Build history of the part. All positions in model axes, mm. Face numbers are marked on the shaded views. Give positions to 0.01 mm unless a question says otherwise; leave off trailing zeros. Loops run counter-clockwise (first coordinate to the right, second up) from the corner with the lowest first, then second, coordinate; pieces in that order, holes last. Notation, with made-up numbers: M 32,87 L 42,87 A12 cw 42,103 Z; hole C 27.25,-13 d2. An arc over 180 degrees is marked long. Put each result on its own line as item: value.
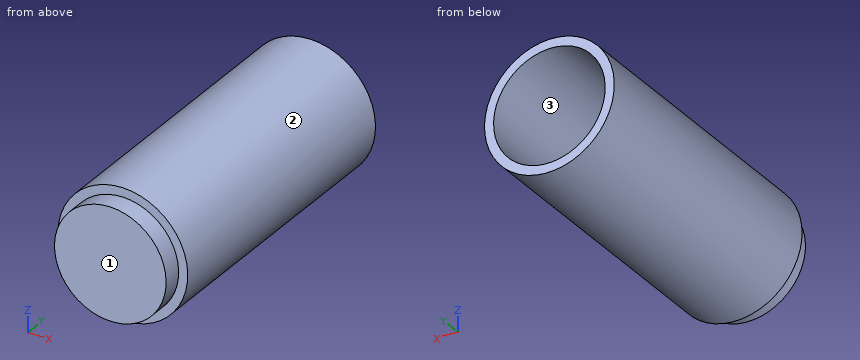
```python
from build123d import *

# Parameters (mm, degrees)
SKETCH1_R           = 50
BOSS_EXTRUDE1_DEPTH = 225
SHELL1_T            = -7
BOSS_EXTRUDE2_START = 15
SKETCH2_R           = 43
BOSS_EXTRUDE2_DEPTH = 15


with BuildPart() as part:
    # Sketch1 → Boss-Extrude1 (new body)
    with BuildSketch(Plane(origin=(0, 0, 0), x_dir=(1, 0, 0), z_dir=(0, 1, 0))):
        with Locations(Location((0, 0, 0), (0, 0, 270))):
            Circle(SKETCH1_R)
    extrude(amount=BOSS_EXTRUDE1_DEPTH)

    # Shell1
    shell1_openings = [part.faces().sort_by_distance(p)[0] for p in [
        (0, 225, 0),
    ]]
    offset(amount=SHELL1_T, openings=shell1_openings, kind=Kind.INTERSECTION)

    # Sketch2 → Boss-Extrude2 (add)
    with BuildSketch(Plane.XZ.offset(BOSS_EXTRUDE2_START)):
        with Locations(Location((0, 0, 0), (0, 0, 90))):
            Circle(SKETCH2_R)
    extrude(amount=-BOSS_EXTRUDE2_DEPTH)


solid = part.part
```
Q1. Slice it at A-A (x = 0). List the corners of the cut face in (y, z).
Here are the results:
outline: M -15,-43 L 0,-43 L 0,-50 L 225,-50 L 225,-43 L 7,-43 L 7,43 L 225,43 L 225,50 L 0,50 L 0,43 L -15,43 Z
Q2. Slice it at C-C (z = 0). List the corners of the cut face in (x, y), and give its area (3 significant figures).
Here are the results:
outline: M -50,0 L -43,0 L -43,-15 L 43,-15 L 43,0 L 50,0 L 50,225 L 43,225 L 43,7 L -43,7 L -43,225 L -50,225 Z
area: 5,040 mm²
Q3. Mould opens along X. For the marked faces 1, 2 and 3 say: pulls with the +X half, pulls with the -X half, needs draft (parallel to the pull), parting line crosses it, or undercut.
Here are the results:
face 1: needs draft
face 2: parting line crosses it
face 3: undercut
Q4. Probe line 1 (X direction, y = 170.5, z = 0); line 2 (Y direction, x = -16.5, z = -38); line 3 (Y direction, x = 45, z = -3). List the from-to ranges inside material, lowest first. Write a range as from..to.
Here are the results:
line 1: -50..-43, 43..50
line 2: -15..7
line 3: 0..225
Q5. Drop flat-ended pins along their axis: pin 1 Ø5 at (y, z) = (116, -32) entering from +X; pin 2 Ø8 at (x, y) = (13.5, 99.5) entering from +Z; pin 3 Ø2 at (x, y) = (7.5, 124.5) entering from +Z. Give the stop position or say it passes through.
Here are the results:
pin 1: x = 40.37
pin 2: z = 49.09
pin 3: z = 49.58
Q6. Slice it at B-B (y = 31.5). List the corners of the cut face in (x, z), and give its area (3 significant figures).
Here are the results:
outline: C 0,0 d100; hole C 0,0 d86
area: 2,050 mm²
